from build123d import *

# Parameters (mm, degrees)
F2_R            = 12.5
F3_DEPTH        = 20.001
F3_COPIES_COUNT = 4


# Not quite as in the source:
# - a pattern or mirror of a feature is missing from the dataset's text; its kind, count and spacing are read off the source's solid


with BuildPart() as f1:
    # F0 (on Front) → F1 (revolve)
    with BuildSketch(Plane.XZ):
        Polygon((-100, 37.5), (0, 37.5), (0, 90), (-20, 90), (-20, 47.5), (-100, 47.5), align=None)
    revolve(axis=Axis((-86.3388044803, 0, 0), (-1, 0, 0)))

    # F2 (on face) → F3 (cut, through all)
    with BuildSketch(Plane(origin=(-20, 0, 0), x_dir=(0, -1, 0), z_dir=(-1, 0, 0))):
        with Locations((0, 75)):
            Circle(F2_R)
    f3 = extrude(amount=-F3_DEPTH, mode=Mode.SUBTRACT)

    # F3_copies: F3 ×4 about axis
    f3_copies_axis = Axis((0, 0, 0), (1, 0, 0))
    for i in range(1, F3_COPIES_COUNT):
        add(f3.rotate(f3_copies_axis, i * 360 / F3_COPIES_COUNT), mode=Mode.SUBTRACT)


solid = f1.part
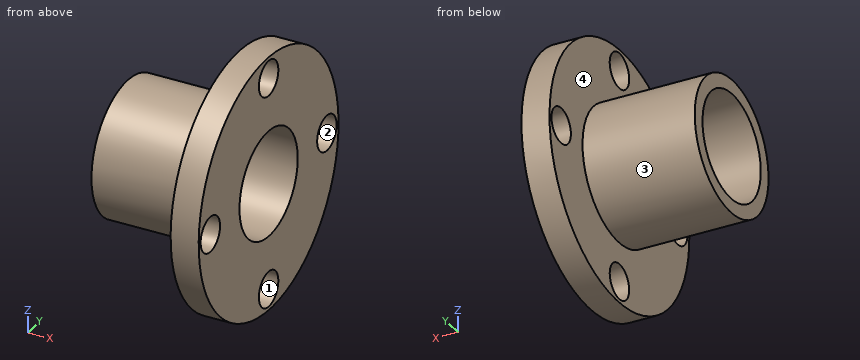
The listing builds one solid part. Answer for the finished solid, in the listing's coordinates (mm). Face numbers are marked on the shaded views. Give positions to 0.01 mm unless a question says otherwise; leave off trailing zeros. Loops run counter-clockwise (first coordinate to the right, second up) from the corner with the lowest first, then second, coordinate; pieces in that order, holes last. Notation, with made-up numbers: (16.25, 69.5) - (41.25, 69.5) arc R25 cw to (41.25, 104.5) - close; hole circle Ø11 at (58, 5). An arc over 180 degrees is marked (long way). Write each question's results on one line, items separated by ' | '.
1. For a pull along Z with two mould halves and no side action, classify the marked faces 1, 2, 3 and 4 as +Z half, -Z half, draft (parallel to the pull), parting line (faces both ways), or undercut.
Resolved:
face 1: undercut | face 2: undercut | face 3: parting line | face 4: draft
2. Find section D-D, the plane z = 31. Write down the section's boundary in (x, y), then the cut area to 3 significant figures.
Resolved:
outline: (-100, -35.99) - (-20, -35.99) - (-20, -84.49) - (0, -84.49) - (0, -21.1) - (-100, -21.1) - close; (-100, 21.1) - (0, 21.1) - (0, 84.49) - (-20, 84.49) - (-20, 35.99) - (-100, 35.99) - close | area: 4,920 mm^2
3. Find section C-C, the plane x = -58. Write down the section's boundary in (y, z).
Resolved:
outline: circle Ø95 at (0, 0); hole circle Ø75 at (0, 0)
4. Find section A-A, the plane y = 0. Write down the section's boundary in (x, z), then the cut area to 3 significant figures.
Resolved:
outline: (-100, -47.5) - (-20, -47.5) - (-20, -62.5) - (0, -62.5) - (0, -37.5) - (-100, -37.5) - close; (-100, 37.5) - (0, 37.5) - (0, 62.5) - (-20, 62.5) - (-20, 47.5) - (-100, 47.5) - close; (-20, -90) - (0, -90) - (0, -87.5) - (-20, -87.5) - close; (-20, 87.5) - (0, 87.5) - (0, 90) - (-20, 90) - close | area: 2,700 mm^2
5. Flat-ended cylindrical pins translate along their axes: P1, Ø1.5, axis at x = -55, y = -3.5, coming from the +Z side; P2, Ø1, axis at x = -59.5, z = -7.5, coming from the -Y side; P3, Ø12, axis at x = -62.5, y = -43.5, coming from the +Z side. Find the tip coordinate at first contact, or state that the pin passes through.
Resolved:
P1: stops at z = 47.42 | P2: stops at y = -46.98 | P3: stops at z = 29.15
6. Consider probe 1 along Y at (x, z) = (-4.5, 0); probe 2 along X at (y, z) = (79.5, -37); probe 3 along Z at (x, y) = (-73.5, -10). Determine where each line is inside the solid, lowest interval first. Write a range as from..to.
Resolved:
probe 1: y = -90..-87.5, -62.5..-37.5, 37.5..62.5, 87.5..90 | probe 2: x = -20..0 | probe 3: z = -46.44..-36.14, 36.14..46.44
